from build123d import *

# Parameters (mm, degrees)
EXTRUDE_1_DEPTH      = 2.5
EXTRUDE_2_DEPTH      = 1
EXTRUDE_2_DEPTH_BACK = 3.5
SKETCH_4_R           = 1.5
CUT_EXTRUDE_1_DEPTH  = 14.5
SKETCH_7_R           = 1
SKETCH_7_R_2         = 0.75
CUT_EXTRUDE_4_DEPTH  = 3
SKETCH_8_R           = 4.75
EXTRUDE_3_DEPTH      = 1.5
EXTRUDE_3_TAPER      = 23
SKETCH_9_R           = 3.25
CUT_EXTRUDE_5_DEPTH  = 3
SKETCH_10_R          = 3.75
CUT_EXTRUDE_6_DEPTH  = 2


with BuildPart() as part:
    # ｽｹｯﾁ1 → ﾎﾞｽ - 押し出し1 (new body)
    with BuildSketch(Plane(origin=(0, 0, 0), x_dir=(1, 0, 0), z_dir=(0, 1, 0))):
        with BuildLine():
            Line((27.647942003, 6.286100267), (-0.344309679, 3.633724101))
            ThreePointArc((-0.344309679, 3.633724101), (-3.65, 0), (-0.344309679, -3.633724101))
            Line((-0.344309679, -3.633724101), (27.647942003, -6.286100267))
            ThreePointArc((27.647942003, -6.286100267), (35.25, 0), (27.647942003, 6.286100267))
        make_face()
    extrude(amount=EXTRUDE_1_DEPTH)

    # ｽｹｯﾁ2 → ﾎﾞｽ - 押し出し2 (add, two sides)
    with BuildSketch(Plane(origin=(0, 2.5, 0), x_dir=(1, 0, 0), z_dir=(0, 1, 0))) as extrude_2_sk:
        with BuildLine():
            Line((27.647942003, 6.286100267), (20.35, 5.594591501))
            Line((20.35, 5.594591501), (20.35, -5.594591501))
            Line((20.35, -5.594591501), (27.647942003, -6.286100267))
            Line((27.647942003, -6.286100267), (28.85, -6.4))
            Line((28.85, -6.4), (29.836801685, -6.323466014))
            ThreePointArc((29.836801685, -6.323466014), (35.25, 0), (29.836801685, 6.323466014))
            Line((29.836801685, 6.323466014), (28.85, 6.4))
            Line((28.85, 6.4), (27.647942003, 6.286100267))
        make_face()
    extrude(amount=EXTRUDE_2_DEPTH)
    extrude(extrude_2_sk.sketch, amount=-EXTRUDE_2_DEPTH_BACK)

    # ｽｹｯﾁ4 → ｶｯﾄ - 押し出し1 (cut)
    with BuildSketch(Plane(origin=(0, 3.5, 0), x_dir=(1, 0, 0), z_dir=(0, 1, 0))):
        with Locations(Location((28.85, 0, 0), (0, 0, 270))):
            Circle(SKETCH_4_R)
    extrude(amount=-CUT_EXTRUDE_1_DEPTH, mode=Mode.SUBTRACT)

    # ｽｹｯﾁ7 → ｶｯﾄ - 押し出し4 (cut)
    with BuildSketch(Plane(origin=(0, 2.5, 0), x_dir=(1, 0, 0), z_dir=(0, 1, 0))):
        with Locations((57.7, 0)):
            Circle(SKETCH_7_R)
        with Locations(Location((15.204795613, 0, 0), (0, 0, 270))):
            Circle(SKETCH_7_R)
        with Locations((54.7, 0)):
            Circle(SKETCH_7_R)
        with Locations((51.7, 0)):
            Circle(SKETCH_7_R)
        with Locations((48.7, 0)):
            Circle(SKETCH_7_R)
        with Locations((45.7, 0)):
            Circle(SKETCH_7_R)
        with Locations(Location((12.204795613, 0, 0), (0, 0, 270))):
            Circle(SKETCH_7_R_2)
        with Locations(Location((9.204795613, 0, 0), (0, 0, 270))):
            Circle(SKETCH_7_R_2)
        with Locations(Location((6.204795613, 0, 0), (0, 0, 270))):
            Circle(SKETCH_7_R_2)
        with Locations(Location((3.204795613, 0, 0), (0, 0, 270))):
            Circle(SKETCH_7_R_2)
        with Locations(Location((0.204795613, 0, 0), (0, 0, 270))):
            Circle(SKETCH_7_R)
    extrude(amount=-CUT_EXTRUDE_4_DEPTH, mode=Mode.SUBTRACT)

    # ｽｹｯﾁ8 → ﾎﾞｽ - 押し出し3 (add)
    with BuildSketch(Plane(origin=(0, -1, 0), x_dir=(-1, 0, 0), z_dir=(0, -1, 0))):
        with Locations((-28.85, 0)):
            Circle(SKETCH_8_R)
    extrude(amount=EXTRUDE_3_DEPTH, taper=EXTRUDE_3_TAPER)

    # ｽｹｯﾁ9 → ｶｯﾄ - 押し出し5 (cut)
    with BuildSketch(Plane(origin=(0, -2.5, 0), x_dir=(-1, 0, 0), z_dir=(0, -1, 0))):
        with Locations(Location((-28.85, 0, 0), (0, 0, 90))):
            Circle(SKETCH_9_R)
    extrude(amount=-CUT_EXTRUDE_5_DEPTH, mode=Mode.SUBTRACT)

    # ｽｹｯﾁ10 → ｶｯﾄ - 押し出し6 (cut)
    with BuildSketch(Plane(origin=(0, 3.5, 0), x_dir=(1, 0, 0), z_dir=(0, 1, 0))):
        with Locations(Location((28.85, 0, 0), (0, 0, 270))):
            Circle(SKETCH_10_R)
    extrude(amount=-CUT_EXTRUDE_6_DEPTH, mode=Mode.SUBTRACT)


solid = part.part
Verification items for the finished model (mm, model axes). A direction names the side the tool comes from. Coordinates: 2 decimals unless noted, no trailing zeros. Write each loop counter-clockwise with the first axis right and the second up, starting at its lowest first coordinate (ties: lowest second). Pieces come first, ordered by that corner, then holes. Notation, with made-up numbers: M 36,27.5 L 69,27.5 A33 cw 69,59.5 Z; hole C 55.25,32.5 d6. An arc over 180 degrees is marked long. One line per question, with ' | ' between items.
1) Sectioned sample at A-A on z = 0. State how many separate pieces and enclosed holes the cut face has, then the cut area to 3 significant figures.
Solutions:
separate pieces: 8 | enclosed holes: 0 | area: 77.8 mm^2
2) Access from +Z, -Z, +X, -X, +Y, -Y to the whole of each face (thin tool, end or side, straight path). Record for faces 4 (the face through (20.35, 3, 0)), 5 (the face through (8, 0, 0)), 6 (the face through (25.19, 2.51, -0.81)), 7 (the face through (27, 0.5, -1)).
Solutions:
face 4: +Z, -Z, -X, +Y | face 5: +Z, -Z, -X, -Y | face 6: +Y | face 7: -Y
3) Material ranges on L1, parallel to Y at x = 13.5, z = 2; L2, parallel to Y at x = 31, z = 4.75; L3, parallel to Z at x = 27.5, y = 1, recorded low to high.
Solutions:
L1: 0 to 2.5 | L2: -1 to 3.5 | L3: -6.27 to -0.65, 0.65 to 6.27
4) Release check for a two-part mould opening along Z. For faces 1 (the face through (24, -1, -3)), 2 (the face through (31.59, -1.02, -1.75)), 3 (the face through (29.35, -0.49, -6.36)) record: +Z half, -Z half, draft (parallel to the pull), parting line (faces both ways), or undercut.
Solutions:
face 1: draft | face 2: undercut | face 3: -Z half
5) Sectioned sample at B-B on x = 19.5. Record the cut outline in (y, z).
Solutions:
outline: M 0,-5.51 L 2.5,-5.51 L 2.5,5.51 L 0,5.51 Z
6) Depth check by flat-ended pin: pin 1 Ø3 at (x, y) = (13, 0.5) entering from +Z; pin 2 Ø1.2 at (x, z) = (12.2, 0) entering from +Y; pin 3 Ø3.5 at (x, z) = (9.5, 0.5) entering from +Y; pin 4 Ø3 at (x, z) = (0.2, 0) entering from -Y. Enter the tip coordinate at first touch or a pass-through.
Solutions:
pin 1: z = 5.04 | pin 2: through | pin 3: y = 2.5 | pin 4: y = 0
